from build123d import *

# Parameters (mm, degrees)
ESQUISSE1_R        = 30
BOSS_EXTRU_1_DEPTH = 2
ESQUISSE2_W        = 14.2
ESQUISSE2_H        = 8.2
ESQUISSE2_W_2      = 10.2
ESQUISSE2_H_2      = 4.2
BOSS_EXTRU_2_DEPTH = 15


with BuildPart() as part:
    # Esquisse1 → Boss.-Extru.1 (new body)
    with BuildSketch(Plane(origin=(0, 0, 0), x_dir=(1, 0, 0), z_dir=(0, 1, 0))):
        with Locations(Location((0, 0, 0), (0, 0, 270))):
            Circle(ESQUISSE1_R)
    extrude(amount=BOSS_EXTRU_1_DEPTH)

    # Esquisse2 → Boss.-Extru.2 (add)
    with BuildSketch(Plane(origin=(0, 2, 0), x_dir=(1, 0, 0), z_dir=(0, 1, 0))):
        Rectangle(ESQUISSE2_W, ESQUISSE2_H)
        Rectangle(ESQUISSE2_W_2, ESQUISSE2_H_2, mode=Mode.SUBTRACT)
    extrude(amount=BOSS_EXTRU_2_DEPTH)


solid = part.part
Design review of the part built by this model. Coordinates are the model's own, in mm. A direction names the side the tool comes from. Round coordinates to 2 decimals unless told otherwise and drop trailing zeros. Loops run counter-clockwise (first coordinate to the right, second up) from the corner with the lowest first, then second, coordinate; pieces in that order, holes last. Notation, with made-up numbers: (1, -16.5) - (9, -16.5) arc R30 ccw to (9, 12.5) - close; hole circle Ø3 at (27, 69). An arc over 180 degrees is marked (long way). One line per item, written item: value. Start each with the question number.
1) For faces 1 (the flat face through (0, 9, -2.1)), 2 (the flat face through (-7.1, 9, 0)), 3 (the flat face through (0, 9, -4.1)), 4 (the flat face through (0, 9, 4.1)), 5 (the cylindrical face through (1.32, 0.99, -29.97)), list the 3-axis set-ups (+Z, -Z, +X, -X, +Y, -Y) from which the entire face can be reached by the end or side of a thin tool; tool diameter is ignored.
2) Insertion check: pin 1 Ø8 at (y, z) = (15, -4) entering from +X; pin 2 Ø5 at (x, z) = (-17.5, -4.5) entering from -Y; pin 3 Ø7 at (x, y) = (0, 9) entering from -Z; pin 4 Ø8 at (x, y) = (2, 7.5) entering from +Z. Each pin has a flat end and moves straight along its axis. Give the tip position at first contact, or say it passes through.
3) To check wall thickness, follow L1, parallel to Y at x = 13, z = 11; L2, parallel to X at y = 8, z = 3.5; L3, parallel to Z at x = 0, y = 8.5. State the ranges of each line that lie inside material, in increasing order. Write a range as from..to.
4) Consider section D-D on z = -15. Give the boundary of the cut face in (x, y).
5) Consider section A-A on y = 2.75. Give the boundary of the cut face in (x, z).
6) Consider section B-B on z = 0. Give the boundary of the cut face in (x, y), then the cut area to 3 significant figures.
7) Draft analysis for pull direction X (two halves, no side actions). For faces 6 (the flat face through (-5.1, 9, 0)), 7 (the flat face through (0, 17, -3)), 8 (the flat face through (7.1, 9, 0)), state which applies: +X half, -X half, draft (parallel to the pull), parting line (faces both ways), or undercut.
8) Consider section C-C on x = 0. Give the boundary of the cut face in (y, z).
Reported:
1. face 1: +Y
1. face 2: +Z, -Z, -X, +Y
1. face 3: -Z, +X, -X, +Y
1. face 4: +Z, +X, -X, +Y
1. face 5: +Y, -Y
2. pin 1: stops at x = 7.1
2. pin 2: stops at y = 0
2. pin 3: stops at z = -4.1
2. pin 4: stops at z = 4.1
3. L1: y = 0..2
3. L2: x = -7.1..7.1
3. L3: z = -4.1..-2.1, 2.1..4.1
4. outline: (-25.98, 0) - (25.98, 0) - (25.98, 2) - (-25.98, 2) - close
5. outline: (-7.1, -4.1) - (7.1, -4.1) - (7.1, 4.1) - (-7.1, 4.1) - close; hole (-5.1, -2.1) - (5.1, -2.1) - (5.1, 2.1) - (-5.1, 2.1) - close
6. outline: (-30, 0) - (30, 0) - (30, 2) - (7.1, 2) - (7.1, 17) - (5.1, 17) - (5.1, 2) - (-5.1, 2) - (-5.1, 17) - (-7.1, 17) - (-7.1, 2) - (-30, 2) - close
6. area: 180 mm^2
7. face 6: undercut
7. face 7: draft
7. face 8: +X half
8. outline: (0, -30) - (2, -30) - (2, -4.1) - (17, -4.1) - (17, -2.1) - (2, -2.1) - (2, 2.1) - (17, 2.1) - (17, 4.1) - (2, 4.1) - (2, 30) - (0, 30) - close
